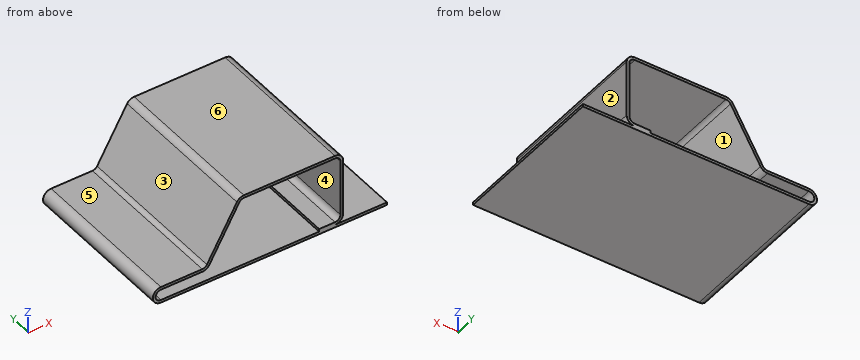
from build123d import *

# Parameters (mm, degrees)
SKETCH2_W = 70
SKETCH2_H = 1.2


with BuildPart() as part:
    # Sweep1: sweep along a path in Sketch4
    with BuildLine(Plane(origin=(0, 0, 0), x_dir=(-1, 0, 0), z_dir=(0, 1, 0))) as sweep1_path:
        Line((0, 0), (100, 0))
        ThreePointArc((100, 0), (103, 3), (100, 6))
        Line((100, 6), (81.732050808, 6))
        ThreePointArc((81.732050808, 6), (80.232050808, 6.401923789), (79.133974596, 7.5))
        Line((79.133974596, 7.5), (65.866025404, 30.480762114))
        ThreePointArc((65.866025404, 30.480762114), (64.767949192, 31.578838325), (63.267949192, 31.980762114))
        Line((63.267949192, 31.980762114), (23, 31.980762114))
        ThreePointArc((23, 31.980762114), (20.878679656, 31.102082457), (20, 28.980762114))
        Line((20, 28.980762114), (20, 4.200762114))
        ThreePointArc((20, 4.200762114), (20.878679656, 2.07944177), (23, 1.200762114))
        Line((23, 1.200762114), (30, 1.200762114))
    # Sketch2 → Sweep1 (sweep)
    with BuildSketch(Plane.YZ):
        Rectangle(SKETCH2_W, SKETCH2_H)
    sweep(path=sweep1_path.line)


solid = part.part
Verification items for the finished model (mm, model axes). Face numbers are marked on the shaded views. A direction names the side the tool comes from. Round coordinates to 2 decimals unless told otherwise and drop trailing zeros. Loops run counter-clockwise (first coordinate to the right, second up) from the corner with the lowest first, then second, coordinate; pieces in that order, holes last. Notation, with made-up numbers: (75, 10.25) - (107, 10.25) arc R34 cw to (107, 43.25) - close; hole circle Ø3 at (5.5, 61.25). An arc over 180 degrees is marked (long way). Write item = value, one per line.
Q1. Sectioned sample at B-B on z = 20.5. Record the boundary of the cut face in (x, y).
Here are the results:
outline = (-72.32, -35) - (-70.94, -35) - (-70.94, 35) - (-72.32, 35) - close; (-20.6, -35) - (-19.4, -35) - (-19.4, 35) - (-20.6, 35) - close
Q2. Depth check by flat-ended pin: pin 1 (6 mm diameter, centred on x = -67, y = -22.5, fed in from +Z); pin 2 (1 mm diameter, centred on y = 4.5, z = 1, fed in from -X); pin 3 (12.5 mm diameter, centred on y = -14.5, z = 20, fed in from -X). Enter the tip coordinate at first touch or a pass-through.
Here are the results:
pin_1 = 32.51
pin_2 = -103.27
pin_3 = -76.22
Q3. Sectioned sample at A-A on x = -97. Record the boundary of the cut face in (y, z).
Here are the results:
outline = (-35, -0.6) - (35, -0.6) - (35, 0.6) - (-35, 0.6) - close; (-35, 5.4) - (35, 5.4) - (35, 6.6) - (-35, 6.6) - close
Q4. Mould release check, pull along X, two halves, no side actions. Record for the marked faces 1, 2 and 3: +X half, -X half, draft (parallel to the pull), parting line (faces both ways), or undercut.
Here are the results:
face_1 = undercut
face_2 = +X half
face_3 = -X half
Q5. Material ranges on L1, parallel to Z at x = -57.5, y = -31; L2, parallel to Z at x = -94.5, y = -24; L3, parallel to X at y = 6, z = 3, recorded low to high.
Here are the results:
L1 = -0.6 to 0.6, 31.38 to 32.58
L2 = -0.6 to 0.6, 5.4 to 6.6
L3 = -103.6 to -102.4, -20.92 to -19.61
Q6. Tool access check on the marked faces 4, 5 and 6. Record the directions out of +Z, -Z, +X, -X, +Y, -Y that give a thin tool (end or side, any length) a straight path to the whole face; none if there is none.
Here are the results:
face_4 = +Y, -Y
face_5 = +Z, -X, +Y, -Y
face_6 = +Z, +X, -X, +Y, -Y
Q7. Sectioned sample at C-C on y = 17.5. Record the boundary of the cut face in (x, z), plus the area to 3 significant figures.
Here are the results:
outline = (-100, -0.6) - (0, -0.6) - (0, 0.6) - (-100, 0.6) arc R2.4 cw to (-100, 5.4) - (-81.73, 5.4) arc R3.6 ccw to (-78.61, 7.2) - (-65.35, 30.18) arc R2.4 cw to (-63.27, 31.38) - (-23, 31.38) arc R2.4 cw to (-20.6, 28.98) - (-20.6, 4.2) arc R2.4 cw to (-23, 1.8) - (-30, 1.8) - (-30, 0.6) - (-23, 0.6) arc R3.6 ccw to (-19.4, 4.2) - (-19.4, 28.98) arc R3.6 ccw to (-23, 32.58) - (-63.27, 32.58) arc R3.6 ccw to (-66.39, 30.78) - (-79.65, 7.8) arc R2.4 cw to (-81.73, 6.6) - (-100, 6.6) arc R3.6 ccw to start
area = 290 mm^2
